```python
from build123d import *

# Parameters (mm, degrees)
SKETCH_1_R      = 2.6
SKETCH_1_R_2    = 2.15
EXTRUDE_1_DEPTH = 3


with BuildPart() as part:
    # 草图1 → 凸台-拉伸1 (new body)
    with BuildSketch(Plane(origin=(0, 0, 0), x_dir=(1, 0, 0), z_dir=(0, 1, 0))):
        Polygon((-75, 290), (-115, 290), (-115, 115), (-290, 115), (-290, 75), (-250, 75), (-250, -75), (-290, -75), (-290, -115), (-115, -115), (-115, -290), (-75, -290), (-75, -250), (75, -250), (75, -290), (115, -290), (115, -115), (290, -115), (290, -75), (250, -75), (250, 75), (290, 75), (290, 115), (115, 115), (115, 290), (75, 290), (75, 250), (-75, 250), align=None)
        with Locations(Location((-105, 280, 0), (0, 0, 270))):
            Circle(SKETCH_1_R, mode=Mode.SUBTRACT)
        with Locations(Location((-47.5, 220, 0), (0, 0, 270))):
            Circle(SKETCH_1_R_2, mode=Mode.SUBTRACT)
        with Locations(Location((-47.5, 245, 0), (0, 0, 270))):
            Circle(SKETCH_1_R_2, mode=Mode.SUBTRACT)
        with Locations(Location((47.5, 220, 0), (0, 0, 270))):
            Circle(SKETCH_1_R_2, mode=Mode.SUBTRACT)
        with Locations(Location((47.5, 245, 0), (0, 0, 270))):
            Circle(SKETCH_1_R_2, mode=Mode.SUBTRACT)
        with Locations(Location((105, 280, 0), (0, 0, 270))):
            Circle(SKETCH_1_R, mode=Mode.SUBTRACT)
        with Locations(Location((44, 105, 0), (0, 0, 270))):
            Circle(SKETCH_1_R, mode=Mode.SUBTRACT)
        with Locations(Location((-37, -105, 0), (0, 0, 270))):
            Circle(SKETCH_1_R, mode=Mode.SUBTRACT)
        with Locations(Location((44, -105, 0), (0, 0, 270))):
            Circle(SKETCH_1_R, mode=Mode.SUBTRACT)
        with Locations(Location((-37, 105, 0), (0, 0, 270))):
            Circle(SKETCH_1_R, mode=Mode.SUBTRACT)
        with Locations(Location((-118, 105, 0), (0, 0, 270))):
            Circle(SKETCH_1_R, mode=Mode.SUBTRACT)
        with Locations(Location((-280, -105, 0), (0, 0, 270))):
            Circle(SKETCH_1_R, mode=Mode.SUBTRACT)
        with Locations(Location((-199, -105, 0), (0, 0, 270))):
            Circle(SKETCH_1_R, mode=Mode.SUBTRACT)
        with Locations(Location((-245, -47.5, 0), (0, 0, 270))):
            Circle(SKETCH_1_R_2, mode=Mode.SUBTRACT)
        with Locations(Location((-220, -47.5, 0), (0, 0, 270))):
            Circle(SKETCH_1_R_2, mode=Mode.SUBTRACT)
        with Locations(Location((-118, -105, 0), (0, 0, 270))):
            Circle(SKETCH_1_R, mode=Mode.SUBTRACT)
        with Locations(Location((-245, 47.5, 0), (0, 0, 270))):
            Circle(SKETCH_1_R_2, mode=Mode.SUBTRACT)
        with Locations(Location((-220, 47.5, 0), (0, 0, 270))):
            Circle(SKETCH_1_R_2, mode=Mode.SUBTRACT)
        with Locations(Location((-280, 105, 0), (0, 0, 270))):
            Circle(SKETCH_1_R, mode=Mode.SUBTRACT)
        with Locations(Location((-199, 105, 0), (0, 0, 270))):
            Circle(SKETCH_1_R, mode=Mode.SUBTRACT)
        with Locations(Location((105, -280, 0), (0, 0, 270))):
            Circle(SKETCH_1_R, mode=Mode.SUBTRACT)
        with Locations(Location((-105, -280, 0), (0, 0, 270))):
            Circle(SKETCH_1_R, mode=Mode.SUBTRACT)
        with Locations(Location((-47.5, -245, 0), (0, 0, 270))):
            Circle(SKETCH_1_R_2, mode=Mode.SUBTRACT)
        with Locations(Location((-47.5, -220, 0), (0, 0, 270))):
            Circle(SKETCH_1_R_2, mode=Mode.SUBTRACT)
        with Locations(Location((47.5, -245, 0), (0, 0, 270))):
            Circle(SKETCH_1_R_2, mode=Mode.SUBTRACT)
        with Locations(Location((47.5, -220, 0), (0, 0, 270))):
            Circle(SKETCH_1_R_2, mode=Mode.SUBTRACT)
        with Locations(Location((280, 105, 0), (0, 0, 270))):
            Circle(SKETCH_1_R, mode=Mode.SUBTRACT)
        with Locations(Location((125, -105, 0), (0, 0, 270))):
            Circle(SKETCH_1_R, mode=Mode.SUBTRACT)
        with Locations(Location((206, -105, 0), (0, 0, 270))):
            Circle(SKETCH_1_R, mode=Mode.SUBTRACT)
        with Locations(Location((280, -105, 0), (0, 0, 270))):
            Circle(SKETCH_1_R, mode=Mode.SUBTRACT)
        with Locations(Location((220, -47.5, 0), (0, 0, 270))):
            Circle(SKETCH_1_R_2, mode=Mode.SUBTRACT)
        with Locations(Location((245, -47.5, 0), (0, 0, 270))):
            Circle(SKETCH_1_R_2, mode=Mode.SUBTRACT)
        with Locations(Location((125, 105, 0), (0, 0, 270))):
            Circle(SKETCH_1_R, mode=Mode.SUBTRACT)
        with Locations(Location((220, 47.5, 0), (0, 0, 270))):
            Circle(SKETCH_1_R_2, mode=Mode.SUBTRACT)
        with Locations(Location((245, 47.5, 0), (0, 0, 270))):
            Circle(SKETCH_1_R_2, mode=Mode.SUBTRACT)
        with Locations(Location((206, 105, 0), (0, 0, 270))):
            Circle(SKETCH_1_R, mode=Mode.SUBTRACT)
    extrude(amount=EXTRUDE_1_DEPTH)


solid = part.part
```
The model under review builds one solid part; all positions refer to its coordinate system, in mm. Give positions to 0.01 mm unless a question says otherwise; leave off trailing zeros. Write each loop counter-clockwise with the first axis right and the second up, starting at its lowest first coordinate (ties: lowest second). Pieces come first, ordered by that corner, then holes. Notation, with made-up numbers: (44.5, 61.5) - (85.5, 61.5) arc R17 ccw to (85.5, 68.5) - close; hole circle Ø4 at (70, 41). An arc over 180 degrees is marked (long way). Answer in a Markdown table with one row per item. Add a question column.
1. We need section B-B on z = -10. Write out the cut boundary in (x, y).
2. We need section C-C on y = 1.85. State how many separate pieces and enclosed holes the cut face has, then the cut area to 3 significant figures.
3. Wall thickness on line 1 along Z through (x, y) = (206, 1.6); line 2 along X through (y, z) = (0.95, -280); line 3 along X through (y, z) = (2.65, -220): over which ranges is each line inside the solid? List them lowest first. Write a range as [from, to].
4. We need section A-A on x = 33. Write out the cut boundary in (y, z), then the cut area to 3 significant figures.
5. Insertion check: P1, Ø0.9, axis at x = -5, y = 1.5, coming from the +Z side. The pin has a flat end and moves straight along its axis. Give the tip position at first contact, or say it passes through.
Ans:
| question | item | result |
|---|---|---|
| 1 | outline | (-250, 0) - (250, 0) - (250, 3) - (-250, 3) - close |
| 2 | separate pieces | 1 |
| 2 | enclosed holes | 36 |
| 2 | area | 189,000 mm^2 |
| 3 | line 1 | z = [-115, -107.6], [-102.4, 102.4], [107.6, 115] |
| 3 | line 2 | x = [-115, -107.6], [-102.4, -75], [75, 102.4], [107.6, 115] |
| 3 | line 3 | x = [-115, -49.65], [-45.35, 45.35], [49.65, 115] |
| 4 | outline | (0, -250) - (3, -250) - (3, 250) - (0, 250) - close |
| 4 | area | 1,500 mm^2 |
| 5 | P1 | stops at z = 250 |
